The model under review builds one solid part; all positions refer to its coordinate system, in mm. Face numbers are marked on the shaded views. A direction names the side the tool comes from. Coordinates: 2 decimals unless noted, no trailing zeros. Order: outer loops, then holes, each group sorted by start corner. A loop starts at its lowest first (then second) coordinate and runs counter-clockwise, first axis right, second up.
Autodesk Inventor part; units mm, degrees
ref_plane "YZ Plane" through (0, 0, 0) normal (1, 0, 0) x (0, 1, 0)
ref_plane "XZ Plane" through (0, 0, 0) normal (0, 1, 0) x (-1, 0, 0)
ref_plane "XY Plane" through (0, 0, 0) normal (0, 0, 1) x (1, 0, 0)
sketch "Sketch1" plane through (0, 0, 0) normal (0, 1, 0) x (-1, 0, 0)
  line L0 (0, 44.45) -> (-22.25, 44.45)
  line L1 (-22.25, 44.45) -> (-66.75, 38.05)
  line L2 (-66.75, 38.05) -> (-89, 38.05)
  line L3 (-89, 0) -> (0, 0)
  line L4 (-89, 35.15) -> (-64.4351, 35.15)
  line L5 (-64.4351, 35.15) -> (-22.0211, 41.25)
  line L6 (-22.0211, 41.25) -> (0, 41.25)
  line L7 (-89, 0) -> (-89, 35.15) construction
  line L8 (-89, 38.05) -> (-89, 35.15)
  line L9 (0, 44.45) -> (0, 41.25)
  line L10 (0, 0) -> (0, 41.25) construction
  dimension "d0" = 88.9
  dimension "d1" = 76.1
  dimension "d2" = 3.2
  dimension "d3" = 2.9
  dimension "d4" = 89
  dimension "d5" = 22.25
  dimension "d6" = 22.25
  dimension "d7" = 3.2
revolve "Revolution1" add sketch "Sketch1" angle 360 about axis through (89, 0, 0) along (-1, 0, 0)
equation "\"d0\" = D"
equation "\"d1\" = D1"
equation "\"d2\" = T"
equation "\"d3\" = T1"
equation "\"d4\" = L"
equation "\"d5\" = 0.25 * L"
equation "\"d6\" = 0.25 * L"
equation "\"d7\" = T"
equation "\"T\" = 3.2"
equation "\"D\" = 88.9"
equation "\"D1\" = 76.1"
equation "\"L\" = 89"
equation "\"T1\" = 2.9"
equation "\"Size_Designation\" = 1.2345"
properties part number "ISO 5251 Concentric reducers DN80 x DN65 3,2" material "Stainless Steel"
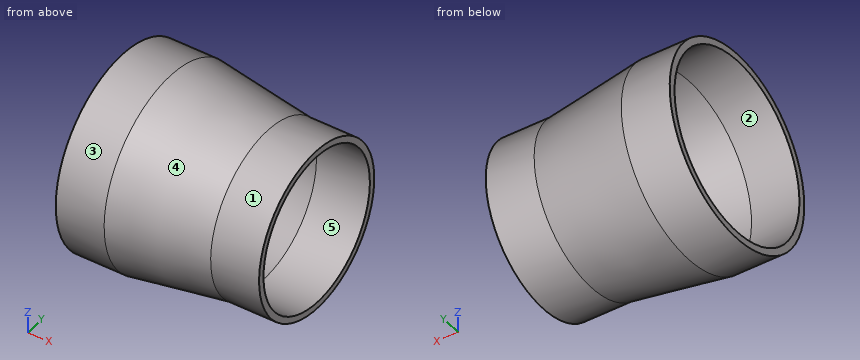
(1) Machinability: for the marked faces 1, 2 and 3, which of the approach directions +Z, -Z, +X, -X, +Y, -Y give a long, thin tool a straight path to every point of the face, cutting with its end or side? Answer none if there is none.
A:
face 1: +X
face 2: -X
face 3: +X, -X
(2) For pin 1 Ø1 at (x, z) = (64, -31) entering from -Y; pin 2 Ø3 at (x, z) = (32, 20.5) entering from +Y; pin 3 Ø5 at (x, z) = (25.5, 25) entering from +Y, all flat-tipped, find the tip position at first contact; note any pin that passes through.
A:
pin 1: stops at y = -23.42
pin 2: stops at y = 38.67
pin 3: stops at y = 37.85
(3) Wall thickness on probe 1 along Y at (x, z) = (83.25, 0); probe 2 along Y at (x, z) = (11.5, 0); probe 3 along Z at (x, y) = (36.5, 14.5): over which ranges is each line inside the solid? List them lowest first.
A:
probe 1: y = -38.05 to -35.15, 35.15 to 38.05
probe 2: y = -44.45 to -41.25, 41.25 to 44.45
probe 3: z = -39.84 to -36.38, 36.38 to 39.84
(4) We need section A-A, the plane z = 0. Write out the cut boundary in (x, y), and give its area (3 significant figures).
A:
outline: (0, -44.45) - (22.25, -44.45) - (66.75, -38.05) - (89, -38.05) - (89, -35.15) - (64.44, -35.15) - (22.02, -41.25) - (0, -41.25) - close; (0, 41.25) - (22.02, 41.25) - (64.44, 35.15) - (89, 35.15) - (89, 38.05) - (66.75, 38.05) - (22.25, 44.45) - (0, 44.45) - close
area: 558 mm2
(5) We need section C-C, the plane x = 82. Write out the cut boundary in (y, z), and give its area (3 significant figures).
A:
outline: circle Ø76.1 at (0, 0); hole circle Ø70.3 at (0, 0)
area: 667 mm2
(6) Draft analysis for pull direction Z (two halves, no side actions). For the marked faces 4 and 5, state which applies: released by +Z, released by -Z, zero draft, split by the parting line, or undercut.
A:
face 4: split by the parting line
face 5: undercut
(7) We need section B-B, the plane x = 19. Write out the cut boundary in (y, z), and give its area (3 significant figures).
A:
outline: circle Ø88.9 at (0, 0); hole circle Ø82.5 at (0, 0)
area: 862 mm2
